```python
from build123d import *

# Parameters (mm, degrees)
BOX062_W          = 5
BOX062_H          = 8
BOX062_DEPTH      = 86
CYLINDER121_R     = 3.6
CYLINDER121_DEPTH = 5
BOX064_W          = 11
BOX064_H          = 5
BOX064_DEPTH      = 14
CYLINDER120_R     = 3.6
CYLINDER120_DEPTH = 5
BOX063_W          = 11
BOX063_H          = 5
BOX063_DEPTH      = 14
TUBE014_R         = 3.6
TUBE014_R_2       = 2
TUBE014_DEPTH     = 2.5
TUBE015_R         = 3.6
TUBE015_R_2       = 2
TUBE015_DEPTH     = 2.5
CYLINDER108_R     = 2
CYLINDER108_DEPTH = 7
CYLINDER107_R     = 2
CYLINDER107_DEPTH = 7
BOX050_W          = 32
BOX050_H          = 10
BOX050_DEPTH      = 4
CHAMFER002_SIZE   = 3


with BuildPart() as cube062:
    # Box062 → Box062 (new body)
    with BuildSketch(Plane(origin=(-5.5, 8, 8), x_dir=(0, 1, 0), z_dir=(1, 0, 0))):
        with Locations((2.5, 4)):
            Rectangle(BOX062_W, BOX062_H)
    extrude(amount=BOX062_DEPTH)


with BuildPart() as cylinder121:
    # Cylinder121 → Cylinder121 (new body)
    with BuildSketch(Plane(origin=(75, -73, 0), x_dir=(0, 0, -1), z_dir=(0, -1, 0))):
        Circle(CYLINDER121_R)
    extrude(amount=CYLINDER121_DEPTH)


with BuildPart() as cut066:
    # Box064 → Box064 (new body)
    with BuildSketch(Plane(origin=(69.5, -78, -6), x_dir=(1, 0, 0), z_dir=(0, 0, 1))):
        with Locations((5.5, 2.5)):
            Rectangle(BOX064_W, BOX064_H)
    extrude(amount=BOX064_DEPTH)

    # Cut066: cut Cylinder121
    add(cylinder121.part, mode=Mode.SUBTRACT)


with BuildPart() as cut066_1:
    # Cut066 placement: moved
    add(cut066.part.moved(Location((0, 86, 0))))


with BuildPart() as cylinder120:
    # Cylinder120 → Cylinder120 (new body)
    with BuildSketch(Plane(origin=(0, -73, 0), x_dir=(0, 0, -1), z_dir=(0, -1, 0))):
        Circle(CYLINDER120_R)
    extrude(amount=CYLINDER120_DEPTH)


with BuildPart() as cut065:
    # Box063 → Box063 (new body)
    with BuildSketch(Plane(origin=(-5.5, -78, -6), x_dir=(1, 0, 0), z_dir=(0, 0, 1))):
        with Locations((5.5, 2.5)):
            Rectangle(BOX063_W, BOX063_H)
    extrude(amount=BOX063_DEPTH)

    # Cut065: cut Cylinder120
    add(cylinder120.part, mode=Mode.SUBTRACT)


with BuildPart() as cut065_1:
    # Cut065 placement: moved
    add(cut065.part.moved(Location((0, 86, 0))))


with BuildPart() as tube014:
    # Tube014 → Tube014 (new body)
    with BuildSketch(Plane.XZ.offset(-13)):
        Circle(TUBE014_R)
        Circle(TUBE014_R_2, mode=Mode.SUBTRACT)
    extrude(amount=TUBE014_DEPTH)


with BuildPart() as tube015:
    # Tube015 → Tube015 (new body)
    with BuildSketch(Plane(origin=(75, 13, 0), x_dir=(1, 0, 0), z_dir=(0, -1, 0))):
        Circle(TUBE015_R)
        Circle(TUBE015_R_2, mode=Mode.SUBTRACT)
    extrude(amount=TUBE015_DEPTH)


with BuildPart() as cylinder108:
    # Cylinder108 → Cylinder108 (new body)
    with BuildSketch(Plane(origin=(28, -68, 7), x_dir=(1, 0, 0), z_dir=(0, 0, 1))):
        Circle(CYLINDER108_R)
    extrude(amount=CYLINDER108_DEPTH)


with BuildPart() as fusion053:
    # Cylinder107 → Cylinder107 (new body)
    with BuildSketch(Plane(origin=(48, -68, 7), x_dir=(1, 0, 0), z_dir=(0, 0, 1))):
        Circle(CYLINDER107_R)
    extrude(amount=CYLINDER107_DEPTH)

    # Fusion053: union Cylinder108
    add(cylinder108.part)


with BuildPart() as fusion053_1:
    # Fusion053 placement: moved
    add(fusion053.part.moved(Location((0, 0, 3))))


with BuildPart() as chamfer002:
    # Box050 → Box050 (new body)
    with BuildSketch(Plane(origin=(22, -73, 13), x_dir=(1, 0, 0), z_dir=(0, 0, 1))):
        with Locations((16, 5)):
            Rectangle(BOX050_W, BOX050_H)
    extrude(amount=BOX050_DEPTH)

    # Cut050: cut Fusion053
    add(fusion053_1.part, mode=Mode.SUBTRACT)


with BuildPart() as chamfer002_1:
    # Cut050 placement: moved
    add(chamfer002.part.moved(Location((-0.5, 71, -1))))

    # Fusion104: union Cube062, Cut066, Cut065, Tube014, Tube015
    add(cube062.part)
    add(cut066_1.part)
    add(cut065_1.part)
    add(tube014.part)
    add(tube015.part)

    # Chamfer002
    chamfer002_edges = [chamfer002_1.edges().sort_by_distance(p)[0] for p in [
        (5.5, 10.5, 8),
        (69.5, 10.5, 8),
    ]]
    chamfer(chamfer002_edges, length=CHAMFER002_SIZE)


solid = chamfer002_1.part
```
The listing builds one solid part. Answer for the finished solid, in the listing's coordinates (mm). A direction names the side the tool comes from. Give positions to 0.01 mm unless a question says otherwise; leave off trailing zeros. Order: outer loops, then holes, each group sorted by start corner. A loop starts at its lowest first (then second) coordinate and runs counter-clockwise, first axis right, second up.
1) For faces 1 (the face through (2, 10.5, -2)), 2 (the face through (7, 10.5, 6.5)), 3 (the face through (0, 12, -2)), 4 (the face through (53.5, 3, 14)), 5 (the face through (37, 3, 12)), determine the directions among +Z, -Z, +X, -X, +Y, -Y from which every point of the face is accessible in a straight line to the end or side of a thin tool.
Reported:
face 1: -Y
face 2: -Z, +Y, -Y
face 3: +Y, -Y
face 4: +Z, -Z, +X, -Y
face 5: -Z, +X, -X, -Y
2) Given P1, Ø1.2, axis at y = 3.5, z = 14, coming from the -X side; P2, Ø1.5, axis at y = 2.5, z = 12, coming from the +X side; P3, Ø4.5, axis at x = 27.5, y = 3, coming from the -Z side, each flat-ended and moving along its own axis, determine where each tip first touches the part or whether it passes through.
Reported:
P1: stops at x = 21.5
P2: stops at x = 53.5
P3: stops at z = 12
3) Find section C-C on z = 13.75. Write down the section's boundary in (x, y), then the cut area to 3 significant figures.
Reported:
outline: (-5.5, 8) - (21.5, 8) - (21.5, -2) - (53.5, -2) - (53.5, 8) - (80.5, 8) - (80.5, 13) - (-5.5, 13) - close; hole circle Ø4 at (27.5, 3); hole circle Ø4 at (47.5, 3)
area: 725 mm2
4) Determine the mould class of faces 6 (the face through (21.5, 3, 14)), 7 (the face through (76.908, 11.768, 0.601)), 8 (the face through (75, 11, -6)) for opening direction X: pulls with the +X half, pulls with the -X half, needs draft (parallel to the pull), parting line crosses it, or undercut.
Reported:
face 6: pulls with the -X half
face 7: undercut
face 8: needs draft
5) Find section D-D on x = 0. Write down the section's boundary in (y, z).
Reported:
outline: (8, -6) - (13, -6) - (13, -2) - (10.5, -2) - (10.5, -3.6) - (8, -3.6) - close; (8, 3.6) - (10.5, 3.6) - (10.5, 2) - (13, 2) - (13, 16) - (8, 16) - close
6) Find section A-A on x = 27.5. Write down the section's boundary in (y, z), then the cut area to 3 significant figures.
Reported:
outline: (-2, 12) - (1, 12) - (1, 16) - (-2, 16) - close; (5, 12) - (8, 12) - (8, 8) - (13, 8) - (13, 16) - (5, 16) - close
area: 64.0 mm2
7) Find section B-B on z = 0. Write down the section's boundary in (x, y).
Reported:
outline: (-5.5, 8) - (-3.6, 8) - (-3.6, 10.5) - (-2, 10.5) - (-2, 13) - (-5.5, 13) - close; (2, 10.5) - (3.6, 10.5) - (3.6, 8) - (5.5, 8) - (5.5, 13) - (2, 13) - close; (69.5, 8) - (71.4, 8) - (71.4, 10.5) - (73, 10.5) - (73, 13) - (69.5, 13) - close; (77, 10.5) - (78.6, 10.5) - (78.6, 8) - (80.5, 8) - (80.5, 13) - (77, 13) - close
8) Consider line 1 along X through (y, z) = (8.5, 0); line 2 along X through (y, z) = (3, 14.8); line 3 along Y through (x, z) = (27.5, 12.8). Determine where each line is inside the solid, lowest interval first.
Reported:
line 1: x = -5.5 to -3.6, 3.6 to 5.5, 69.5 to 71.4, 78.6 to 80.5
line 2: x = 21.5 to 25.5, 29.5 to 45.5, 49.5 to 53.5
line 3: y = -2 to 1, 5 to 13
